Answer from the drawing. Dimensions are ordinates in mm from the lowest x, y and z of the part. Give positions to 0.01 mm unless a question says otherwise; leave off trailing zeros. Loops run counter-clockwise (first coordinate to the right, second up) from the corner with the lowest first, then second, coordinate; pieces in that order, holes last.
(1) Find section C-C, the plane z = 19.05. Write down the section's boundary in (x, y), then the cut area to 3 significant figures.
(2) Find section D-D, the plane x = 95.25. Write down the section's boundary in (y, z).
(3) Straight lines are drawn through the part: probe 1 along Z at (x, y) = (95.25, 20); probe 2 along Z at (x, y) = (165, 21.5) (1 decimal); probe 3 along Z at (x, y) = (171.45, 15.25). For each, find the intervals that lie inside material, in ascending order.
(4) Find section A-A, the plane z = 95.25. Write down the section's boundary in (x, y).
(5) Find section B-B, the plane x = 19.05. Write down the section's boundary in (y, z), then the cut area to 3 significant figures.
(6) Each of these flat-tipped pins is pushed along its axis until it touches: P1, Ø16, axis at x = 95.25, z = 19.05, coming from the -Y side; P2, Ø1.5, axis at y = 8.5, z = 55.5, coming from the +X side; P3, Ø6, axis at x = 53, y = 22.5, coming from the +Z side; P4, Ø5, axis at x = 29.5, y = 3.5, coming from the -Z side. Where does it stop, or does it pass through?
(7) Determine the mould class of the marked faces 1, 2 and 3 for opening direction Z: pulls with the +Z half, pulls with the -Z half, needs draft (parallel to the pull), parting line crosses it, or undercut.
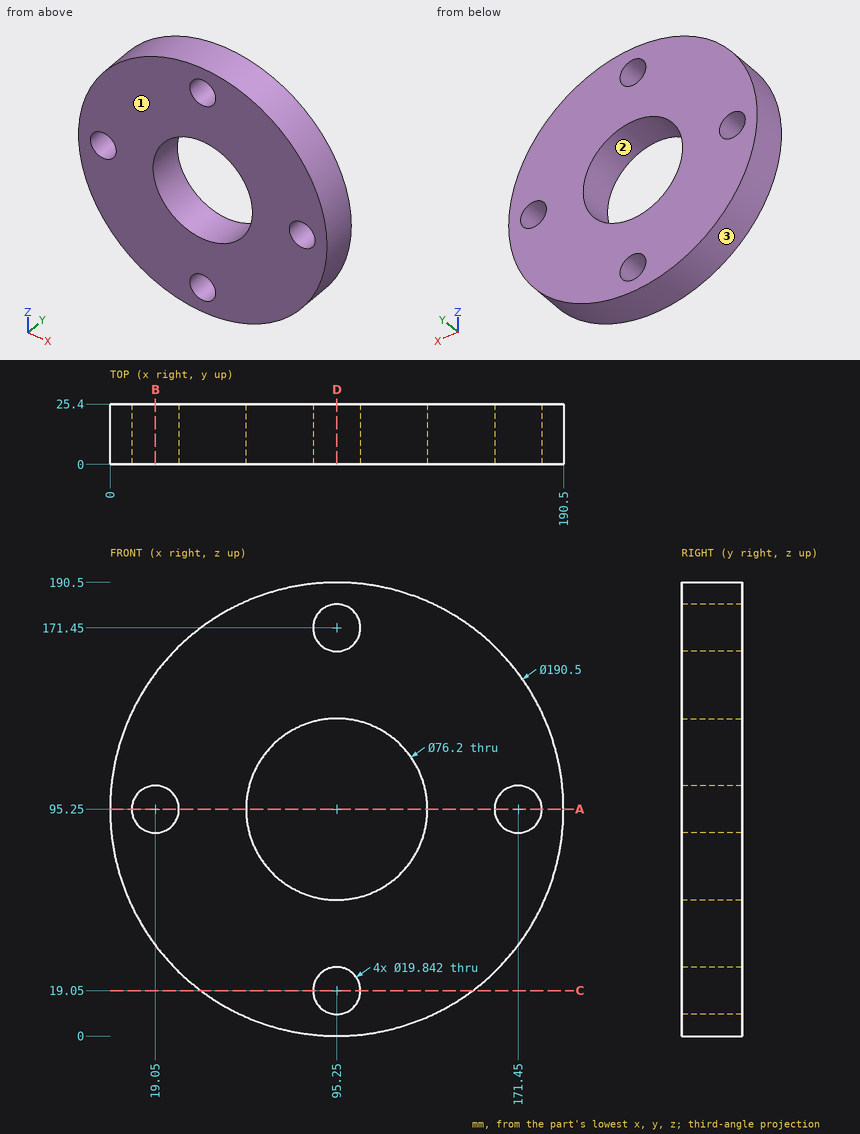
Entries:
1. outline: (38.1, 0) - (85.33, 0) - (85.33, 25.4) - (38.1, 25.4) - close; (105.17, 0) - (152.4, 0) - (152.4, 25.4) - (105.17, 25.4) - close
1. area: 2,400 mm2
2. outline: (0, 0) - (25.4, 0) - (25.4, 9.13) - (0, 9.13) - close; (0, 28.97) - (25.4, 28.97) - (25.4, 57.15) - (0, 57.15) - close; (0, 133.35) - (25.4, 133.35) - (25.4, 161.53) - (0, 161.53) - close; (0, 181.37) - (25.4, 181.37) - (25.4, 190.5) - (0, 190.5) - close
3. probe 1: z = 0 to 9.13, 28.97 to 57.15, 133.35 to 161.53, 181.37 to 190.5
3. probe 2: z = 30.4 to 87.7, 102.8 to 160.1
3. probe 3: z = 38.1 to 85.33, 105.17 to 152.4
4. outline: (0, 0) - (9.13, 0) - (9.13, 25.4) - (0, 25.4) - close; (28.97, 0) - (57.15, 0) - (57.15, 25.4) - (28.97, 25.4) - close; (133.35, 0) - (161.53, 0) - (161.53, 25.4) - (133.35, 25.4) - close; (181.37, 0) - (190.5, 0) - (190.5, 25.4) - (181.37, 25.4) - close
5. outline: (0, 38.1) - (25.4, 38.1) - (25.4, 85.33) - (0, 85.33) - close; (0, 105.17) - (25.4, 105.17) - (25.4, 152.4) - (0, 152.4) - close
5. area: 2,400 mm2
6. P1: passes through
6. P2: stops at x = 182.15
6. P3: stops at z = 182.04
6. P4: stops at z = 24.03
7. face 1: needs draft
7. face 2: undercut
7. face 3: parting line crosses it
